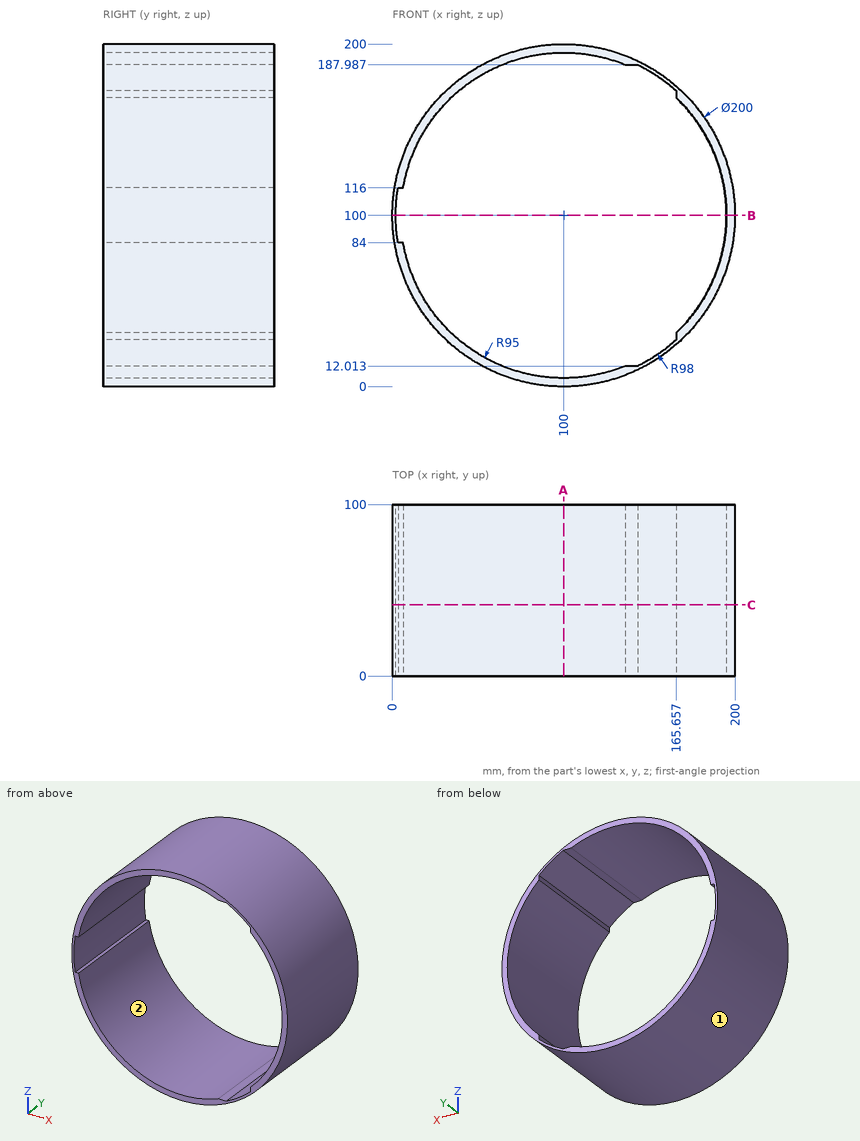
Here's the drawing with two shaded views (mm, measured from the low corner). I have some questions. Give positions to 0.01 mm unless a question says otherwise; leave off trailing zeros. Loops run counter-clockwise (first coordinate to the right, second up) from the corner with the lowest first, then second, coordinate; pieces in that order, holes last. Notation, with made-up numbers: M 51,78 L 74,78 A32 ccw 74,115 Z; hole C -37,66 d4. An arc over 180 degrees is marked long. Answer in a Markdown table with one row per item.
1. Thinking about a two-plate mould opening in Z: for the marked faces 1 and 2, which applies, released by +Z, released by -Z, zero draft, split by the parting line, or undercut?
Taken from the geometry:
| item | result |
|---|---|
| face 1 | split by the parting line |
| face 2 | undercut |
2. For pin 1 Ø2 at (x, y) = (139, 43.5) entering from +Z; pin 2 Ø6 at (x, y) = (140, 37) entering from -Z; pin 3 Ø12 at (y, z) = (68, 51.5) entering from +X; pin 4 Ø5 at (y, z) = (82.5, 101.5) entering from -X, each with a flat end and sliding along its axis, tell me the tip position at first contact or that it passes through.
Taken from the geometry:
| item | result |
|---|---|
| pin 1 | stops at z = 192.5 |
| pin 2 | stops at z = 7.1 |
| pin 3 | stops at x = 190.52 |
| pin 4 | stops at x = 0 |
3. If I drill on line 1 along Z through (x, y) = (102, 66); line 2 along X through (y, z) = (14.5, 143.5) (1 decimal); line 3 along Z through (x, y) = (86, 7) (1 decimal), over which ranges is the centre line in solid material (lowest first)?
Taken from the geometry:
| item | result |
|---|---|
| line 1 | z = 0.02 to 5.02, 194.98 to 199.98 |
| line 2 | x = 10 to 15.5, 184.5 to 190 |
| line 3 | z = 1 to 6, 194 to 199 |
4. Suppose I cut it at C-C on y = 41.5. Write out the boundary of the cut face in (x, z) (1 decimal), plus the area to 3 significant figures.
Taken from the geometry:
| item | result |
|---|---|
| outline | C 100,100 d200; hole M 3.3,84 L 6.4,84 A95 ccw 135.8,12 L 143.2,12 A98 ccw 165.7,27.2 L 165.7,31.3 A95 ccw 165.7,168.7 L 165.7,172.8 A98 ccw 143.2,188 L 135.8,188 A95 ccw 6.4,116 L 3.3,116 A98 ccw Z |
| area | 2,780 mm² |
5. Suppose I cut it at A-A on x = 100. Write out the boundary of the cut face in (y, z).
Taken from the geometry:
| item | result |
|---|---|
| outline | M 0,0 L 100,0 L 100,5 L 0,5 Z; M 0,195 L 100,195 L 100,200 L 0,200 Z |
6. Suppose I cut it at B-B on z = 100. Write out the boundary of the cut face in (x, y), plus the area to 3 significant figures.
Taken from the geometry:
| item | result |
|---|---|
| outline | M 0,0 L 2,0 L 2,100 L 0,100 Z; M 195,0 L 200,0 L 200,100 L 195,100 Z |
| area | 700 mm² |
